Could you check a few things on this model? Use its own coordinates, in mm. Give positions to 0.01 mm unless a question says otherwise; leave off trailing zeros. Write each loop counter-clockwise with the first axis right and the second up, starting at its lowest first coordinate (ties: lowest second). Pieces come first, ordered by that corner, then holes. Notation, with made-up numbers: M 53,70.5 L 99,70.5 A18 ccw 99,89.5 Z; hole C 48,0.5 d7. An arc over 180 degrees is marked long. Use one line per item in the form item = value.
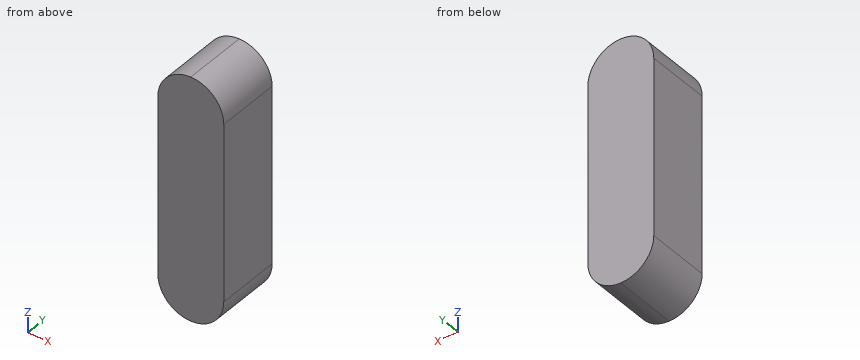
from build123d import *

# Parameters (mm, degrees)
SKETCH1_W      = 6
SKETCH1_H      = 6
EXTRUDE1_DEPTH = 22
FILLET1_R      = 3


with BuildPart() as part:
    # Sketch1 → Extrude1 (new body)
    with BuildSketch(Plane.XY):
        with Locations((3, 4.996296296)):
            Rectangle(SKETCH1_W, SKETCH1_H)
    extrude(amount=EXTRUDE1_DEPTH)

    # Fillet1
    fillet1_edges = [part.edges().sort_by_distance(p)[0] for p in [
        (6, 4.996296296, 22),
        (0, 4.996296296, 22),
        (0, 4.996296296, 0),
        (6, 4.996296296, 0),
    ]]
    fillet(fillet1_edges, radius=FILLET1_R - 0.0001)  # a hair under: the kernel refuses the full size


solid = part.part
1) I want a section at C-C, the plane x = 1.85. Please give me the cut outline in (y, z), plus the area to 3 significant figures.
Checked values:
outline = M 2,0.23 L 8,0.23 L 8,21.77 L 2,21.77 Z
area = 129 mm2
2) For pin 1 Ø3 at (x, y) = (2.5, 5) entering from -Z, with a flat end and sliding along its axis, tell me the tip position at first contact or that it passes through.
Checked values:
pin_1 = 0
3) I want a section at B-B, the plane x = 5.45. Please give me the cut outline in (y, z), plus the area to 3 significant figures.
Checked values:
outline = M 2,1.27 L 8,1.27 L 8,20.73 L 2,20.73 Z
area = 117 mm2
4) If I drill on L1, parallel to Z at x = 2.35, y = 7.2; L2, parallel to Z at x = 1.4, y = 5.3; L3, parallel to X at y = 7.45, z = 19.25, over which ranges is the centre line in solid material (lowest first)?
Checked values:
L1 = 0.07 to 21.93
L2 = 0.46 to 21.54
L3 = 0.01 to 5.99
